The drawing under review shows one solid part. Ordinate dimensions are in mm from its lowest x, y, z. A direction names the side the tool comes from. Coordinates: 2 decimals unless noted, no trailing zeros. Order: outer loops, then holes, each group sorted by start corner. A loop starts at its lowest first (then second) coordinate and runs counter-clockwise, first axis right, second up. Notation, with made-up numbers: (61.25, 80.5) - (94.25, 80.5) arc R13 ccw to (94.25, 104.5) - close; hole circle Ø11 at (41, 67). An arc over 180 degrees is marked (long way). Answer in a Markdown table with one row per item.
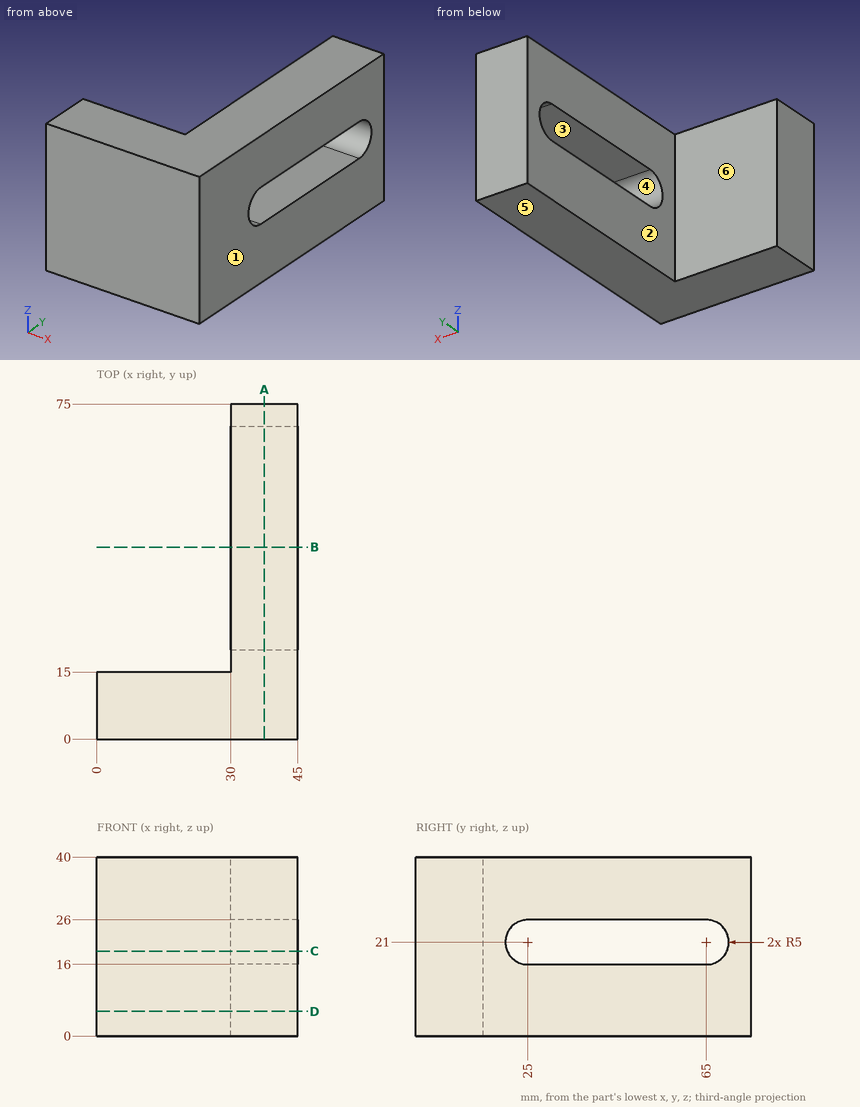
Item 1: To check wall thickness, follow line 1 (Z direction, x = 39.5, y = 55.5); line 2 (Y direction, x = 5.5, z = 11); line 3 (X direction, y = 42, z = 28). State the ranges of each line that lie inside material, in increasing order. Write a range as from..to.
Check values:
| item | result |
|---|---|
| line 1 | 0..16, 26..40 |
| line 2 | 0..15 |
| line 3 | 30..45 |
Item 2: We need section D-D, the plane z = 5.5. Write out the cut boundary in (x, y), then the cut area to 4 significant figures.
Check values:
| item | result |
|---|---|
| outline | (0, 0) - (45, 0) - (45, 75) - (30, 75) - (30, 15) - (0, 15) - close |
| area | 1,575 mm^2 |
Item 3: We need section C-C, the plane z = 19. Write out the cut boundary in (x, y), then the cut area to 3 significant figures.
Check values:
| item | result |
|---|---|
| outline | (0, 0) - (45, 0) - (45, 20.42) - (30, 20.42) - (30, 15) - (0, 15) - close; (30, 69.58) - (45, 69.58) - (45, 75) - (30, 75) - close |
| area | 838 mm^2 |
Item 4: We need section B-B, the plane y = 43. Write out the cut boundary in (x, z), then the cut area to 3 significant figures.
Check values:
| item | result |
|---|---|
| outline | (30, 0) - (45, 0) - (45, 16) - (30, 16) - close; (30, 26) - (45, 26) - (45, 40) - (30, 40) - close |
| area | 450 mm^2 |
Item 5: Tool access review of the marked faces 1, 2 and 3: name each direction out of +Z, -Z, +X, -X, +Y, -Y from which nothing blocks a thin tool from reaching the whole face with its end or side.
Check values:
| item | result |
|---|---|
| face 1 | +Z, -Z, +X, +Y, -Y |
| face 2 | +Z, -Z, -X, +Y |
| face 3 | +X, -X |
Item 6: Mouldability with a two-part tool opening along Y and no side actions: class the marked faces 4, 5 and 6 as +Y half, -Y half, draft (parallel to the pull), parting line (faces both ways), or undercut.
Check values:
| item | result |
|---|---|
| face 4 | undercut |
| face 5 | draft |
| face 6 | +Y half |
Item 7: We need section A-A, the plane x = 37.5. Write out the cut boundary in (y, z), then the cut area to 3 significant figures.
Check values:
| item | result |
|---|---|
| outline | (0, 0) - (75, 0) - (75, 40) - (0, 40) - close; hole (25, 16) - (65, 16) arc R5 ccw to (65, 26) - (25, 26) arc R5 ccw to start |
| area | 2,520 mm^2 |
Item 8: Clearance check with a flat-ended pin moving along its axis: pin 1 Ø9 at (x, z) = (18, 17) entering from +Y. State where the tip first meets the part, or that it passes through.
Check values:
| item | result |
|---|---|
| pin 1 | y = 15 |
